Autodesk Inventor part; units mm, degrees
ref_plane "Work Plane1" through (-497, -256, -240) normal (-1, 0, 0) x (0, 0, 1)
ref_plane "Work Plane2" through (-697, -256, -240) normal (-1, 0, 0) x (0, 0, 1)
ref_plane "Work Plane3" through (-497, -256, -240) normal (-1, 0, 0) x (0, 0, 1)
sketch "Sketch1" plane through (0, 0, 0) normal (1, 0, 0) x (0, 1, 0)
  circle A0 centre (0, 0) radius 6
  dimension "d0" = 12
extrude "Extrusion1" add sketch "Sketch1" along normal blind 10
sketch "Sketch2" plane through (0, 0, 0) normal (-1, 0, 0) x (0, 0, 1)
  circle A0 centre (0, 0) radius 6
ref_plane "Work Plane1" through (-497, -256, -240) normal (-1, 0, 0) x (0, 0, 1)
ref_plane "Work Plane2" through (-697, -256, -240) normal (-1, 0, 0) x (0, 0, 1)
ref_plane "Work Plane3" through (-497, -256, -240) normal (-1, 0, 0) x (0, 0, 1)
ref_plane "Work Plane5" through (-481.5, -422.4955, -226.2332) normal (1, 0, 0) x (0, 0.3162, 0.9487)
extrude "Extrusion3" add sketch "Sketch2" along normal up to surface (481.5 mm away)
sketch "Sketch3" plane through (-481.5, 0, 0) normal (-1, 0, 0) x (0, 0, 1)
  circle A0 centre (0, 0) radius 6
  point P0 (0, 0)
ref_plane "Work Plane6" through (-500.5, -12.5, -12.5) normal (-1, 0, 0) x (0, 0, 1)
extrude "Extrusion4" add sketch "Sketch3" along normal up to surface (19 mm away)
properties part number "12MM_X_AXIS_SHAFT"
Source: CAD feature listing. Evaluate the final solid. Frame: model axes, mm. Round coordinates to 2 decimals unless told otherwise and drop trailing zeros. Loops run counter-clockwise (first coordinate to the right, second up) from the corner with the lowest first, then second, coordinate; pieces in that order, holes last.
Q1. Section A-A, the plane x = -336. Return loops of the section in (y, z), plus the area to 3 significant figures.
Q2. Section C-C, the plane y = -3.5. Return loops of the section in (x, z).
Q3. First-contact query: P1, Ø2, axis at x = -358.5, y = -1.5, coming from the +Z side; P2, Ø1, axis at x = -417.5, y = 1.5, coming from the +Z side; P3, Ø1, axis at x = -278, z = -4.5, coming from the -Y side. Flat tips, straight axial feed; report the tip coordinate or a pass-through.
Q4. Ray query, line 1 (Z direction, x = -295.5, y = -1); line 2 (Z direction, x = -311.5, y = -0.5); line 3 (Y direction, x = -286, z = -0.25). Return the intervals inside material, ascending.
Q5. Section B-B, the plane z = -3.75. Return loops of the section in (x, y).
Solutions:
1. outline: circle Ø12 at (0, 0)
1. area: 113 mm2
2. outline: (-500.5, -4.87) - (10, -4.87) - (10, 4.87) - (-500.5, 4.87) - close
3. P1: stops at z = 5.98
3. P2: stops at z = 5.92
3. P3: stops at y = -4.47
4. line 1: z = -5.92 to 5.92
4. line 2: z = -5.98 to 5.98
4. line 3: y = -5.99 to 5.99
5. outline: (-500.5, -4.68) - (10, -4.68) - (10, 4.68) - (-500.5, 4.68) - close
